For this review, use the dimensioned drawing (mm, ordinates from the lowest corner) and the shaded views. Coordinates: 2 decimals unless noted, no trailing zeros. Loops run counter-clockwise (first coordinate to the right, second up) from the corner with the lowest first, then second, coordinate; pieces in that order, holes last. Notation, with made-up numbers: M 46,57 L 54,57 A17 cw 54,69 Z; hole C -34,63 d1. An arc over 180 degrees is marked long. Write item = value, one per line. Start each with the question number.
Q1. We need section D-D on x = 49. Give the boundary of the cut face in (y, z).
Q2. We need section A-A on x = 20.32. Give the boundary of the cut face in (y, z) (1 decimal), and give its area (3 significant figures).
Q3. Wall thickness on probe 1 along Y at (x, z) = (50.5, 2.5); probe 2 along Y at (x, z) = (215.9, 1.35) (1 decimal): over which ranges is each line inside the solid? List them lowest first.
Q4. We need section C-C on y = 4.25. Give the boundary of the cut face in (x, z).
Q5. We need section B-B on z = 19.25. Give the boundary of the cut face in (x, y).
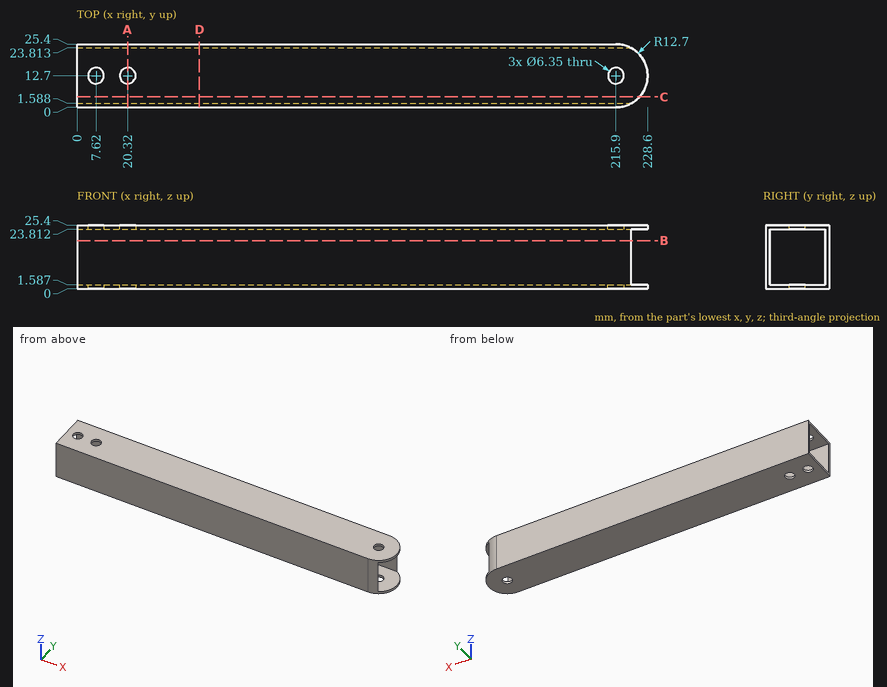
Returned:
q1.outline = M 0,0 L 25.4,0 L 25.4,25.4 L 0,25.4 Z; hole M 1.59,1.59 L 23.81,1.59 L 23.81,23.81 L 1.59,23.81 Z
q2.outline = M 0,0 L 9.5,0 L 9.5,1.6 L 1.6,1.6 L 1.6,23.8 L 9.5,23.8 L 9.5,25.4 L 0,25.4 Z; M 15.9,0 L 25.4,0 L 25.4,25.4 L 15.9,25.4 L 15.9,23.8 L 23.8,23.8 L 23.8,1.6 L 15.9,1.6 Z
q2.area = 131 mm^2
q3.probe_1 = 0 to 1.59, 23.81 to 25.4
q3.probe_2 = 0 to 9.5, 15.9 to 25.4
q4.outline = M 0,0 L 225.38,0 L 225.38,1.59 L 0,1.59 Z; M 0,23.81 L 225.38,23.81 L 225.38,25.4 L 0,25.4 Z
q5.outline = M 0,0 L 215.9,0 A12.7 ccw 222.05,1.59 L 0,1.59 Z; M 0,23.81 L 222.05,23.81 A12.7 ccw 215.9,25.4 L 0,25.4 Z
